from build123d import *

# Parameters (mm, degrees)
F1_DEPTH = 106.426
F2_DEPTH = 25.4


with BuildPart() as f1:
    # F0 (on Front) → F1 (new body)
    with BuildSketch(Plane.XZ):
        Polygon((75.431123, -39.523013), (-71.575209, 55.669609), (-71.575209, -39.523013), align=None)
    extrude(amount=F1_DEPTH)

    # F0 (on Front) → F2 (join)
    with BuildSketch(Plane.XZ):
        Polygon((75.431123, -39.523013), (-71.575209, 55.669609), (-71.575209, -39.523013), align=None)
        Polygon((75.431123, 55.669609), (-71.575209, 55.669609), (75.431123, -39.523013), align=None)
    extrude(amount=F2_DEPTH)


solid = f1.part
Work out the finished part from the listing and answer in its coordinate system (mm). A direction names the side the tool comes from. Give positions to 0.01 mm unless a question says otherwise; leave off trailing zeros. Order: outer loops, then holes, each group sorted by start corner. A loop starts at its lowest first (then second) coordinate and runs counter-clockwise, first axis right, second up. Notation, with made-up numbers: (36.25, 54) -> (41.25, 54) arc R9 cw to (41.25, 65) -> close; hole circle Ø10 at (-7, 49). An arc over 180 degrees is marked (long way). One line per item, written item: value.
Item 1: Find section A-A, the plane x = 24. Give the vertices of the cut face in (y, z), plus the area to 3 significant figures.
Answer sheet:
outline: (-106.43, -39.52) -> (0, -39.52) -> (0, 55.67) -> (-25.4, 55.67) -> (-25.4, -6.22) -> (-106.43, -6.22) -> close
area: 5,120 mm²
Item 2: Flat-ended cylindrical pins translate along their axes: P1, Ø6, axis at y = -95, z = 12.5, coming from the +X side; P2, Ø2, axis at x = -1.5, y = -71.5, coming from the +Z side; P3, Ø1, axis at y = -83, z = -9, coming from the +X side. Find the tip coordinate at first contact, or state that the pin passes through.
Answer sheet:
P1: x = -0.28
P2: z = 10.94
P3: x = 29.07
Item 3: Find section B-B, the plane y = -70. Give the vertices of the cut face in (x, z).
Answer sheet:
outline: (-71.58, -39.52) -> (75.43, -39.52) -> (-71.58, 55.67) -> close
Item 4: Straight lines are drawn through the part: probe 1 along Y at (x, z) = (58.5, -27); probe 2 along Z at (x, y) = (-29, -52); probe 3 along Z at (x, y) = (1, -57). For each, find the intervals that lie inside material, in ascending order.
Answer sheet:
probe 1: -25.4 to 0
probe 2: -39.52 to 28.1
probe 3: -39.52 to 8.67
Item 5: Find section C-C, the plane z = 40. Give the vertices of the cut face in (x, y), plus the area to 3 significant figures.
Answer sheet:
outline: (-71.58, -106.43) -> (-47.38, -106.43) -> (-47.38, -25.4) -> (75.43, -25.4) -> (75.43, 0) -> (-71.58, 0) -> close
area: 5,690 mm²
Item 6: A tool of negligible diameter and unlimited length cuts with its end or side. For faces 1 (the flat face through (1, 0, 9)), 2 (the flat face through (34, -25.4, 30)), from which of +Z, -Z, +X, -X, +Y, -Y can it reach the whole face along a straight path? Write none if from no direction.
Answer sheet:
face 1: +Z, -Z, +X, -X, +Y
face 2: +Z, +X, -Y
